The model under review builds one solid part; all positions refer to its coordinate system, in mm. A direction names the side the tool comes from. Round coordinates to 2 decimals unless told otherwise and drop trailing zeros. Write each loop counter-clockwise with the first axis right and the second up, starting at its lowest first coordinate (ties: lowest second). Pieces come first, ordered by that corner, then holes. Notation, with made-up numbers: M 0.5,5.25 L 7.5,5.25 A23 cw 7.5,16.25 Z; hole C -18.75,10 d4. An arc over 180 degrees is marked long. One line per item, written item: value. Start each with the question number.
1) Take a section at B-B, the plane z = 2.75. Write out the cut boundary in (x, y).
2) Wall thickness on probe 1 along Z at (x, y) = (1.9, 0.7); probe 2 along Y at (x, z) = (0.2, 0.5); probe 3 along X at (y, z) = (0.25, 3): over which ranges is each line inside the solid? List them lowest first.
3) For P1, Ø1.4, axis at x = 4.5, z = 0, coming from the +Y side; P2, Ø1.9, axis at x = 0.5, z = 0, coming from the -Y side, all flat-tipped, find the tip position at first contact; note any pin that passes through.
4) Mouldability with a two-part tool opening along Z and no side actions: class faces 1 (the face through (0.38, 0, 1.44)), 2 (the face through (4.71, 0, 1.46)), 3 (the face through (0.89, 0, 1.46)), 4 (the face through (0, 0.19, 0)) as +Z half, -Z half, draft (parallel to the pull), parting line (faces both ways), or undercut.
5) Take a section at D-D, the plane y = 1.1. Write out the cut boundary in (x, z).
6) Take a section at C-C, the plane x = 2.8. Write out the cut boundary in (y, z), and give its area (3 significant figures).
7) Tool access review of faces 5 (the face through (5.1, -0.19, 0)), 6 (the face through (3, 1.54, 4)), 7 (the face through (5.1, 0.19, 0)), 8 (the face through (4.22, 0, 1.44)): name each direction out of +Z, -Z, +X, -X, +Y, -Y from which nothing blocks a thin tool from reaching the whole face with its end or side.
8) Take a section at A-A, the plane z = 0. Write out the cut boundary in (x, y).
from build123d import *

# Parameters (mm, degrees)
PAD_DEPTH    = 3.7
PAD001_DEPTH = 0.19


with BuildPart() as pad:
    # Sketch → Pad (new body)
    with BuildSketch(Plane.XY.offset(2.5)):
        Polygon((1.11, 1.54), (3.97, 1.54), (4.54, 0), (4.4, -0.77), (0.68, -0.77), (0.54, 0), align=None)
    extrude(amount=PAD_DEPTH)


with BuildPart() as to_92s_2_wide:
    # Sketch001 → Pad001 (new body, symmetric)
    with BuildSketch(Plane.XZ):
        Polygon((0.25, -2.46), (-0.25, -2.46), (-0.25, 0.5), (1.02, 2.4), (1.02, 3.04), (1.52, 3.04), (1.52, 2.4), (0.25, 0.5), align=None)
        Polygon((3.56, 3.04), (4.06, 3.04), (4.06, 2.4), (5.37, 0.5), (5.37, -2.46), (4.87, -2.46), (4.87, 0.5), (3.56, 2.4), align=None)
    extrude(amount=PAD001_DEPTH, both=True)

    add(pad.part)


solid = to_92s_2_wide.part
Checked values:
1. outline: M 0.54,0 L 0.68,-0.77 L 4.4,-0.77 L 4.54,0 L 3.97,1.54 L 1.11,1.54 Z
2. probe 1: z = 2.5 to 6.2
2. probe 2: y = -0.19 to 0.19
2. probe 3: x = 0.63 to 4.45
3. P1: stops at y = 0.19
3. P2: stops at y = -0.19
4. face 1: undercut
4. face 2: undercut
4. face 3: -Z half
4. face 4: draft
5. outline: M 0.95,2.5 L 4.13,2.5 L 4.13,6.2 L 0.95,6.2 Z
6. outline: M -0.77,2.5 L 1.54,2.5 L 1.54,6.2 L -0.77,6.2 Z
6. area: 8.55 mm2
7. face 5: -Z, +X, -X, -Y
7. face 6: +Z, -Z, +X, -X, +Y
7. face 7: -Z, +X, -X, +Y
7. face 8: -Z, +Y, -Y
8. outline: M -0.25,-0.19 L 0.25,-0.19 L 0.25,0.19 L -0.25,0.19 Z; M 4.87,-0.19 L 5.37,-0.19 L 5.37,0.19 L 4.87,0.19 Z
